For this review, take the finished solid that the model builds, in its own axes (mm). A direction names the side the tool comes from. Round coordinates to 2 decimals unless told otherwise and drop trailing zeros. Order: outer loops, then holes, each group sorted by start corner. A loop starts at its lowest first (then second) coordinate and runs counter-clockwise, first axis right, second up. Notation, with made-up numbers: M 85,-35.5 L 124,-35.5 A22 ccw 124,-19.5 Z; hole C 74.5,-1 d8. An arc over 180 degrees is marked long. Use a Markdown table: item, result.
from build123d import *

# Parameters (mm, degrees)
BOSS_EXTRUDE1_DEPTH     = 45
SKETCH2_R               = 3
SKETCH2_W               = 66
SKETCH2_H               = 48.8
CUT_EXTRUDE1_DEPTH      = 60.804765696
CUT_EXTRUDE2_DEPTH      = 59.92546139
CUT_EXTRUDE2_DEPTH_BACK = 59.92546139
SKETCH3_R               = 2


with BuildPart() as part:
    # Sketch1 → Boss-Extrude1 (new, symmetric)
    with BuildSketch(Plane(origin=(0, 0, 0), x_dir=(0, 0, -1), z_dir=(1, 0, 0))):
        Polygon((-38.1, 0), (0, 0), (0, 12), (-2, 12), (-2, 2), (-38.1, 2), align=None)
    extrude(amount=BOSS_EXTRUDE1_DEPTH, both=True)

    # Sketch2 → Cut-Extrude1 (cut, through all)
    with BuildSketch(Plane(origin=(0, 2, 0), x_dir=(1, 0, 0), z_dir=(0, 1, 0))):
        with Locations(Location((37.5, -11.5, 0), (0, 0, 270))):
            Circle(SKETCH2_R)
        with Locations(Location((37.5, -28.5, 0), (0, 0, 90))):
            Circle(SKETCH2_R)
        with Locations(Location((-37.5, -11.5, 0), (0, 0, 90))):
            Circle(SKETCH2_R)
        with Locations(Location((-37.5, -28.5, 0), (0, 0, 270))):
            Circle(SKETCH2_R)
        with Locations((0, -26.4)):
            Rectangle(SKETCH2_W, SKETCH2_H)
    extrude(amount=-CUT_EXTRUDE1_DEPTH, mode=Mode.SUBTRACT)

    # Sketch3 → Cut-Extrude2 (cut, two sides: drawn at the far end of the back side and taken through both)
    with BuildSketch(Plane.XY.offset(2).offset(-CUT_EXTRUDE2_DEPTH_BACK)):
        with Locations((-39, 7)):
            Circle(SKETCH3_R)
        with Locations(Location((39, 7, 0), (0, 0, 90))):
            Circle(SKETCH3_R)
    extrude(amount=CUT_EXTRUDE2_DEPTH + CUT_EXTRUDE2_DEPTH_BACK, mode=Mode.SUBTRACT)


solid = part.part
Q1. Add section A-A (z = 20). Write out the cut boundary in (x, y).
Determined:
| item | result |
|---|---|
| outline | M -45,0 L -33,0 L -33,2 L -45,2 Z; M 33,0 L 45,0 L 45,2 L 33,2 Z |
Q2. Clearance check with flat-ended pins moving along their axes: pin 1 (2 mm diameter, centred on x = -29, y = 7.5, fed in from +Z); pin 2 (3.5 mm diameter, centred on x = -39, y = 7, fed in from -Z); pin 3 (6 mm diameter, centred on x = 37.5, z = 23.5, fed in from +Y). State where each tip first meets the part, or that it passes through.
Determined:
| item | result |
|---|---|
| pin 1 | stops at z = 2 |
| pin 2 | passes through |
| pin 3 | stops at y = 2 |
Q3. Add section D-D (x = 39). Write out the cut boundary in (y, z), then the cut area to 3 significant figures.
Determined:
| item | result |
|---|---|
| outline | M 0,0 L 5,0 L 5,2 L 2,2 L 2,8.9 L 0,8.9 Z; M 0,14.1 L 2,14.1 L 2,25.9 L 0,25.9 Z; M 0,31.1 L 2,31.1 L 2,38.1 L 0,38.1 Z; M 9,0 L 12,0 L 12,2 L 9,2 Z |
| area | 67.4 mm^2 |
Q4. Draft analysis for pull direction Y (two halves, no side actions). For faces 1 (the flat face through (45, 1, 16)), 2 (the cylindrical face through (-41, 7, 1)), 3 (the flat face through (1, 12, 1)), state which applies: pulls with the +Y half, pulls with the -Y half, needs draft (parallel to the pull), parting line crosses it, or undercut.
Determined:
| item | result |
|---|---|
| face 1 | needs draft |
| face 2 | undercut |
| face 3 | pulls with the +Y half |
Q5. Add section C-C (z = 28.5). Write out the cut boundary in (x, y), then the cut area to 3 significant figures.
Determined:
| item | result |
|---|---|
| outline | M -45,0 L -40.5,0 L -40.5,2 L -45,2 Z; M -34.5,0 L -33,0 L -33,2 L -34.5,2 Z; M 33,0 L 34.5,0 L 34.5,2 L 33,2 Z; M 40.5,0 L 45,0 L 45,2 L 40.5,2 Z |
| area | 24.0 mm^2 |
Q6. Add section B-B (y = 7). Write out the cut boundary in (x, z), then the cut area to 3 significant figures.
Determined:
| item | result |
|---|---|
| outline | M -45,0 L -41,0 L -41,2 L -45,2 Z; M -37,0 L 37,0 L 37,2 L -37,2 Z; M 41,0 L 45,0 L 45,2 L 41,2 Z |
| area | 164 mm^2 |
Q7. Wall thickness on line 1 along X through (y, z) = (0.8, 28.5); line 2 along X through (y, z) = (7, 0.85); line 3 along Z through (x, y) = (-18.5, 2.75): over which ranges is each line inside the solid? List them lowest first. Write a range as [from, to].
Determined:
| item | result |
|---|---|
| line 1 | x = [-45, -40.5], [-34.5, -33], [33, 34.5], [40.5, 45] |
| line 2 | x = [-45, -41], [-37, 37], [41, 45] |
| line 3 | z = [0, 2] |
Q8. Machinability: for faces 4 (the flat face through (-39, 2, 20)), 5 (the cylindrical face through (35.47, 1.01, 30.71)), 6 (the flat face through (-33, 1, 20)), which of the approach directions +Z, -Z, +X, -X, +Y, -Y give a long, thin tool a straight path to every point of the face, cutting with its end or side? Answer none if there is none.
Determined:
| item | result |
|---|---|
| face 4 | +Z, +X, -X, +Y |
| face 5 | +Y, -Y |
| face 6 | +Z, +Y, -Y |
